Geometry check sheet. Reference: the model listing, model coordinates, mm. Face numbers are marked on the shaded views. A direction names the side the tool comes from. Round coordinates to 2 decimals unless told otherwise and drop trailing zeros. Order: outer loops, then holes, each group sorted by start corner. A loop starts at its lowest first (then second) coordinate and runs counter-clockwise, first axis right, second up.
(1) Cross-section at B-B on z = 17. Enter the section's corners in (x, y).
(2) Cross-section at D-D on y = -17. Enter the section's corners in (x, z).
(3) Cross-section at C-C on x = 25. Enter the section's corners in (y, z).
(4) Thickness scan on L1, parallel to Z at x = 41.5, y = -5; L2, parallel to Y at x = 39, z = 17; L3, parallel to X at y = -20, z = 19. Record the ranges inside material, lowest first.
(5) Cross-section at A-A on y = -3.25. Enter the section's corners in (x, z), and give its area (3 significant figures).
(6) Set-up check for the marked faces 1, 2 and 3: record each of +Z, -Z, +X, -X, +Y, -Y from which the full face is reachable in a straight line by a thin tool's end or side.
(7) Gauge pin test, flat end, axial feed: P1, Ø4, axis at x = 45.5, y = -7, coming from the +Z side. Record the tip position at first contact, or that the pin passes through.
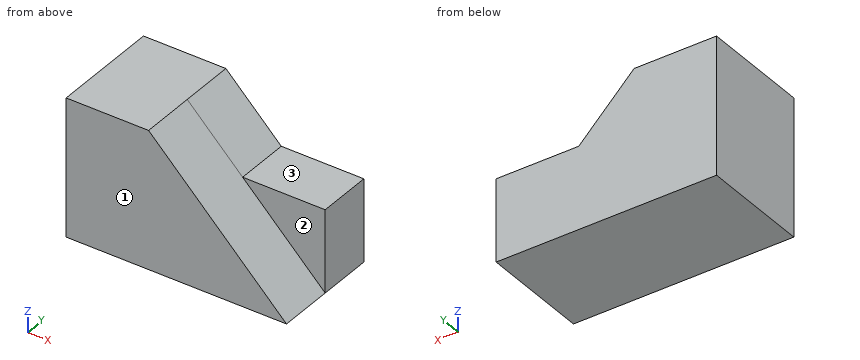
from build123d import *

# Parameters (mm, degrees)
F0_W     = 50.8
F0_H     = 31.75
F1_DEPTH = 25.4
F3_DEPTH = 12.7
F5_DEPTH = 12.7
F7_DEPTH = 12.701


with BuildPart() as f1:
    # F0 (on Front) → F1 (new body)
    with BuildSketch(Plane.XZ):
        with Locations((25.4, 15.875)):
            Rectangle(F0_W, F0_H)
    extrude(amount=F1_DEPTH)

    # F2 (on Front) → F3 (cut)
    with BuildSketch(Plane.XZ):
        Polygon((31.426101923, 5.7290680707), (38.6526212096, -0.4363064363), (50.3639169037, 0), (50.3639169037, 5.7290680707), align=None)
    extrude(amount=-F3_DEPTH, mode=Mode.SUBTRACT)

    # F4 (on face) → F5 (cut)
    with BuildSketch(Plane.XZ.offset(25.4)):
        Polygon((50.8, 31.75), (18.997348845, 31.75), (50.8, 0), align=None)
    extrude(amount=-F5_DEPTH, mode=Mode.SUBTRACT)

    # F6 (on face) → F7 (cut, through all)
    with BuildSketch(Plane.XZ.offset(12.7)):
        Polygon((31.7711477736, 18.997348845), (50.8, 18.997348845), (50.8, 31.75), (18.997348845, 31.75), align=None)
    extrude(amount=-F7_DEPTH, mode=Mode.SUBTRACT)


solid = f1.part
Found:
1. outline: (0, -25.4) - (33.77, -25.4) - (33.77, -12.7) - (50.8, -12.7) - (50.8, 0) - (0, 0) - close
2. outline: (0, 0) - (50.8, 0) - (19, 31.75) - (0, 31.75) - close
3. outline: (-25.4, 0) - (0, 0) - (0, 25.76) - (-25.4, 25.76) - close
4. L1: z = 0 to 19
4. L2: y = -12.7 to 0
4. L3: x = 0 to 31.77
5. outline: (0, 0) - (50.8, 0) - (50.8, 19) - (31.77, 19) - (19, 31.75) - (0, 31.75) - close
5. area: 1,290 mm2
6. face 1: +Z, -Z, +X, -X, -Y
6. face 2: +Z, +X, -Y
6. face 3: +Z, +X, +Y, -Y
7. P1: stops at z = 19
